Design review of the part built by this model. Coordinates are the model's own, in mm. Face numbers are marked on the shaded views. A direction names the side the tool comes from. Give positions to 0.01 mm unless a question says otherwise; leave off trailing zeros. Loops run counter-clockwise (first coordinate to the right, second up) from the corner with the lowest first, then second, coordinate; pieces in that order, holes last.
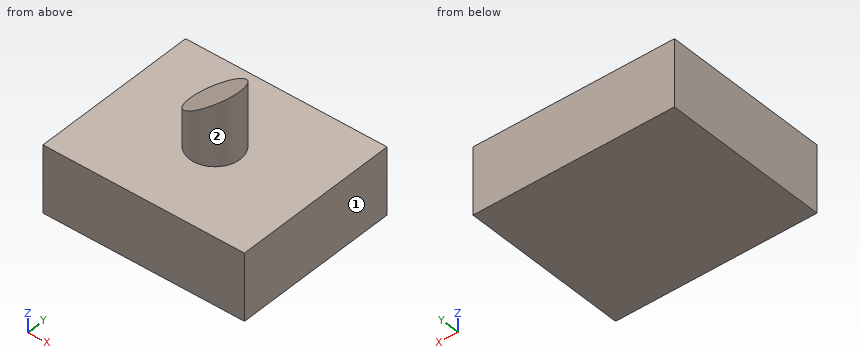
from build123d import *

# Parameters (mm, degrees)
F0_W     = 76.2
F0_H     = 63.5
F1_DEPTH = 25.4
F2_R     = 9.525
F3_DEPTH = 25.4
F5_DEPTH = 19.05


with BuildPart() as f1:
    # F0 (on Top) → F1 (new body)
    with BuildSketch(Plane.XY):
        Rectangle(F0_W, F0_H)
    extrude(amount=F1_DEPTH)

    # F2 (on face) → F3 (join)
    with BuildSketch(Plane.XY.offset(25.4)):
        Circle(F2_R)
    extrude(amount=F3_DEPTH)

    # F4 (on Front) → F5 (cut, symmetric)
    with BuildSketch(Plane.XZ):
        Polygon((9.525, 50.8), (-9.525, 50.8), (-9.525, 38.1), align=None)
    extrude(amount=F5_DEPTH, both=True, mode=Mode.SUBTRACT)


solid = f1.part
Q1. Take a section at B-B (x = 3.5). Give the boundary of the cut face in (y, z), plus the area to 3 significant figures.
Results:
outline: (-31.75, 0) - (31.75, 0) - (31.75, 25.4) - (8.86, 25.4) - (8.86, 46.78) - (-8.86, 46.78) - (-8.86, 25.4) - (-31.75, 25.4) - close
area: 1,990 mm2
Q2. Wall thickness on line 1 (Z direction, x = 28, y = -7); line 2 (Y direction, x = 7, z = 32.5); line 3 (X direction, y = 7.5, z = 43) (3 decimals): over which ranges is each line inside the solid? List them lowest first.
Results:
line 1: z = 0 to 25.4
line 2: y = -6.46 to 6.46
line 3: x = -2.175 to 5.872
Q3. Insertion check: pin 1 (10 mm diameter, centred on x = 4, z = 31.5, fed in from +Y) (3 decimals). The pin has a flat end and moves straight along its axis. Give the tip position at first contact, or say it passes through.
Results:
pin 1: stops at y = 9.525
Q4. Tool access review of the marked faces 1 and 2: name each direction out of +Z, -Z, +X, -X, +Y, -Y from which nothing blocks a thin tool from reaching the whole face with its end or side.
Results:
face 1: +Z, -Z, +X, +Y, -Y
face 2: +Z
Q5. Take a section at C-C (z = 30.5). Give the boundary of the cut face in (x, y) (3 decimals).
Results:
outline: circle Ø19.05 at (0, 0)
Q6. Take a section at A-A (y = 0). Give the boundary of the cut face in (x, z) (3 decimals).
Results:
outline: (-38.1, 0) - (38.1, 0) - (38.1, 25.4) - (9.525, 25.4) - (9.525, 50.8) - (-9.525, 38.1) - (-9.525, 25.4) - (-38.1, 25.4) - close
Q7. Take a section at D-D (x = -30). Give the boundary of the cut face in (y, z), plus the area to 3 significant figures.
Results:
outline: (-31.75, 0) - (31.75, 0) - (31.75, 25.4) - (-31.75, 25.4) - close
area: 1,610 mm2
